Can you work these out from the model? Positions are in its coordinate system, mm. A direction names the side the tool comes from. Coordinates: 2 decimals unless noted, no trailing zeros. Put each result on its own line as item: value. Start each with the question number.
Item 1: Please list where these lines run through material, in increasing order: L1, parallel to Y at x = -1.5, z = 248; L2, parallel to X at y = -46, z = 151; L3, parallel to Z at x = -177, y = 118. Write a range as from..to.
Item 2: For faces 1 (the flat face through (-193, 107, 128)), 2 (the flat face through (-194, 105, 128)), 3 (the flat face through (191.67, 141.66, 256.34)), 4 (the flat face through (-171, -137, 128)), 5 (the flat face through (155, -143, 128)), which set-ups out of +Z, -Z, +X, -X, +Y, -Y let a thin tool reach every point of the face, with its end or its side?
Item 3: We'd pull the mould along Y, two halves only. Please class faces 6 (the flat face through (-191.67, -141.66, 256.34)), 7 (the flat face through (193.049, -140.192, 256.339)), 8 (the flat face through (-155, -144, 128)): pulls with the +Y half, pulls with the -Y half, needs draft (parallel to the pull), parting line crosses it, or undercut.
Item 4: Will these pins go through, and if not, where does the flat tip stop? P1, Ø10.5, axis at x = -195.5, z = 124.5, coming from the +Y side; P2, Ø1.5, axis at x = -25.5, z = 119.5, coming from the -Y side; P3, Ø1, axis at y = -65, z = 87.5, coming from the -X side.
```python
from build123d import *

# Parameters (mm, degrees)
F0_W      = 372
F0_H      = 272
F1_DEPTH  = 15
F2_W      = 372
F2_H      = 272
F3_DEPTH  = 2
F5_DEPTH  = 226
F7_DEPTH  = 2
F9_DEPTH  = 23
F11_DEPTH = 2
F12_W     = 370
F12_H     = 270
F13_DEPTH = 268
F15_DEPTH = 13
F17_DEPTH = 13
F18_R     = 2


with BuildPart() as f1:
    # F0 (on Top) → F1 (new body)
    with BuildSketch(Plane.XY):
        Rectangle(F0_W, F0_H)
    extrude(amount=F1_DEPTH)

    # F2 (on face) → F3 (join)
    with BuildSketch(Plane.XY.offset(15)):
        with BuildLine():
            Line((-190, -150), (190, -150))
            ThreePointArc((190, -150), (197.0710678119, -147.0710678119), (200, -140))
            Line((200, -140), (200, 140))
            ThreePointArc((200, 140), (197.0710678119, 147.0710678119), (190, 150))
            Line((190, 150), (-190, 150))
            ThreePointArc((-190, 150), (-197.0710678119, 147.0710678119), (-200, 140))
            Line((-200, 140), (-200, -140))
            ThreePointArc((-200, -140), (-197.0710678119, -147.0710678119), (-190, -150))
        make_face()
        Rectangle(F2_W, F2_H, mode=Mode.SUBTRACT)
        Rectangle(F2_W, F2_H)
    extrude(amount=F3_DEPTH)

    # F4 (on face) → F5 (join)
    with BuildSketch(Plane.XY.offset(17)):
        Polygon((157, -137), (187, -137), (187, -107), (200, -107), (200, -105), (187, -105), (187, 105), (200, 105), (200, 107), (187, 107), (187, 137), (157, 137), (157, 150), (155, 150), (155, 137), (-155, 137), (-155, 150), (-157, 150), (-157, 137), (-187, 137), (-187, 107), (-200, 107), (-200, 105), (-187, 105), (-187, -105), (-200, -105), (-200, -107), (-187, -107), (-187, -137), (-157, -137), (-157, -150), (-155, -150), (-155, -137), (155, -137), (155, -150), (157, -150), align=None)
    extrude(amount=F5_DEPTH)

    # F6 (on face) → F7 (join)
    with BuildSketch(Plane.XY.offset(243)):
        with BuildLine():
            Line((190, 150), (-190, 150))
            ThreePointArc((-190, 150), (-197.0710678119, 147.0710678119), (-200, 140))
            Line((-200, 140), (-200, -140))
            ThreePointArc((-200, -140), (-197.0710678119, -147.0710678119), (-190, -150))
            Line((-190, -150), (190, -150))
            ThreePointArc((190, -150), (197.0710678119, -147.0710678119), (200, -140))
            Line((200, -140), (200, 140))
            ThreePointArc((200, 140), (197.0710678119, 147.0710678119), (190, 150))
        make_face()
    extrude(amount=F7_DEPTH)

    # F8 (on face) → F9 (join)
    with BuildSketch(Plane.XY.offset(245)):
        with BuildLine():
            Line((-185.3079227659, -137), (185.3079227659, -137))
            Line((185.3079227659, -137), (197.8531877713, -146.1909160735))
            ThreePointArc((197.8531877713, -146.1909160735), (198.4340605379, -145.3727667773), (198.9300207482, -144.5005254622))
            Line((198.9300207482, -144.5005254622), (187, -135.7603498338))
            Line((187, -135.7603498338), (187, 135.7603498338))
            Line((187, 135.7603498338), (198.9300207482, 144.5005254622))
            ThreePointArc((198.9300207482, 144.5005254622), (198.4340605379, 145.3727667773), (197.8531877713, 146.1909160735))
            Line((197.8531877713, 146.1909160735), (185.3079227659, 137))
            Line((185.3079227659, 137), (-185.3079227659, 137))
            Line((-185.3079227659, 137), (-197.8531877713, 146.1909160735))
            ThreePointArc((-197.8531877713, 146.1909160735), (-198.4340605379, 145.3727667773), (-198.9300207482, 144.5005254622))
            Line((-198.9300207482, 144.5005254622), (-187, 135.7603498338))
            Line((-187, 135.7603498338), (-187, -135.7603498338))
            Line((-187, -135.7603498338), (-198.9300207482, -144.5005254622))
            ThreePointArc((-198.9300207482, -144.5005254622), (-198.4340605379, -145.3727667773), (-197.8531877713, -146.1909160735))
            Line((-197.8531877713, -146.1909160735), (-185.3079227659, -137))
        make_face()
    extrude(amount=F9_DEPTH)

    # F10 (on face) → F11 (join)
    with BuildSketch(Plane.XY.offset(268)):
        with BuildLine():
            Line((-190, -150), (190, -150))
            ThreePointArc((190, -150), (197.0710678119, -147.0710678119), (200, -140))
            Line((200, -140), (200, 140))
            ThreePointArc((200, 140), (197.0710678119, 147.0710678119), (190, 150))
            Line((190, 150), (-190, 150))
            ThreePointArc((-190, 150), (-197.0710678119, 147.0710678119), (-200, 140))
            Line((-200, 140), (-200, -140))
            ThreePointArc((-200, -140), (-197.0710678119, -147.0710678119), (-190, -150))
        make_face()
    extrude(amount=F11_DEPTH)

    # F12 (on face) → F13 (cut)
    with BuildSketch(Plane.XY.offset(270)):
        Rectangle(F12_W, F12_H)
    extrude(amount=-F13_DEPTH, mode=Mode.SUBTRACT)

    # F14 (on face) → F15 (join, through all)
    with BuildSketch(Plane(origin=(-187, 0, 0), x_dir=(0, -1, 0), z_dir=(-1, 0, 0))):
        with BuildLine():
            Line((-63, 211), (63, 211))
            ThreePointArc((63, 211), (65.8284271247, 212.1715728753), (67, 215))
            Line((67, 215), (67, 243))
            Line((67, 243), (65, 243))
            Line((65, 243), (65, 215))
            ThreePointArc((65, 215), (64.4142135624, 213.5857864376), (63, 213))
            Line((63, 213), (-63, 213))
            ThreePointArc((-63, 213), (-64.4142135624, 213.5857864376), (-65, 215))
            Line((-65, 215), (-65, 243))
            Line((-65, 243), (-67, 243))
            Line((-67, 243), (-67, 215))
            ThreePointArc((-67, 215), (-65.8284271247, 212.1715728753), (-63, 211))
        make_face()
    extrude(amount=F15_DEPTH)

    # F16 (on face) → F17 (join, through all)
    with BuildSketch(Plane.YZ.offset(187)):
        with BuildLine():
            ThreePointArc((63, 211), (65.8284271247, 212.1715728753), (67, 215))
            Line((67, 215), (67, 243))
            Line((67, 243), (65, 243))
            Line((65, 243), (65, 215))
            ThreePointArc((65, 215), (64.4142135624, 213.5857864376), (63, 213))
            Line((63, 213), (-63, 213))
            ThreePointArc((-63, 213), (-64.4142135624, 213.5857864376), (-65, 215))
            Line((-65, 215), (-65, 243))
            Line((-65, 243), (-67, 243))
            Line((-67, 243), (-67, 215))
            ThreePointArc((-67, 215), (-65.8284271247, 212.1715728753), (-63, 211))
            Line((-63, 211), (63, 211))
        make_face()
    extrude(amount=F17_DEPTH)

    # F18
    f18_edges = [f1.edges().sort_by_distance(p)[0] for p in [
        (-185, -135, 136),
        (185, -135, 136),
        (185, 135, 136),
        (0, 135, 2),
        (185, 0, 2),
        (0, -135, 2),
        (-185, 0, 2),
        (-185, 135, 136),
        (187, -137, 130),
        (187, 137, 130),
        (-187, 137, 130),
        (-187, -137, 130),
        (186, 0, 0),
        (0, 136, 0),
        (186, 136, 7.5),
        (0, -136, 0),
        (186, -136, 7.5),
        (-186, -136, 7.5),
        (-186, 0, 0),
        (-186, 136, 7.5),
    ]]
    fillet(f18_edges, radius=F18_R)


solid = f1.part
```
Solutions:
1. L1: -137..-135, 135..137
1. L2: -187..-185, 185..187
1. L3: 0..2
2. face 1: -X, +Y
2. face 2: -X
2. face 3: +Y
2. face 4: -X, -Y
2. face 5: -Y
3. face 6: pulls with the -Y half
3. face 7: undercut
3. face 8: needs draft
4. P1: y = 107
4. P2: y = -137
4. P3: x = -187
